Autodesk Fusion 360 part; units mm, degrees
sketch "Excentric Triunghiular Ruleaux + Frame-ul cadrului culisant" plane through (0, 0, 0) normal (1, 0, 0) x (0, 1, 0)
  line L0 (-9.5, 5.4848) -> (0, -10.9697) construction
  line L1 (0, -10.9697) -> (9.5, 5.4848) construction
  line L2 (9.5, 5.4848) -> (-9.5, 5.4848) construction
  arc A0 (0, -10.9697) -> (9.5, 5.4848) centre (-9.5, 5.4848) ccw
  arc A1 (-9.5, 5.4848) -> (0, -10.9697) centre (9.5, 5.4848) ccw
  arc A2 (9.5, 5.4848) -> (-9.5, 5.4848) centre (0, -10.9697) ccw
  circle A3 centre (0, -6) radius 2.5
  line L3 (-17.5, 8.0303) -> (17.5, 8.0303)
  line L4 (17.5, 8.0303) -> (17.5, -10.9697)
  line L5 (17.5, -10.9697) -> (-17.5, -10.9697)
  line L6 (-17.5, -10.9697) -> (-17.5, 8.0303)
  line L7 (0, 8.0303) -> (0, -10.9697) construction
  line L8 (20, -13.4697) -> (-20, -13.4697)
  line L9 (-20, -13.4697) -> (-20, 10.5303)
  line L10 (-20, 10.5303) -> (20, 10.5303)
  line L11 (20, 10.5303) -> (20, -13.4697)
  line L12 (17.5, -1.4697) -> (0, -1.4697) construction
  dimension "d4" = 19
  dimension "d5" = 5
  dimension "d6" = 35
  dimension "d7" = 19
  dimension "d8" = 6
  dimension "d9" = 17.5
  dimension "d10" = -2.5
extrude "Extrude1" add sketch "Excentric Triunghiular Ruleaux + Frame-ul cadrului culisant" along normal blind 5 contours A0 A1 A2
equation "d9 = ( 35 / 2 ) * 1 mm"
Can you work these out from the model? Positions are in its coordinate system, mm. Coordinates: 2 decimals unless noted, no trailing zeros. Loops run counter-clockwise (first coordinate to the right, second up) from the corner with the lowest first, then second, coordinate; pieces in that order, holes last. Notation, with made-up numbers: (53, -9.5) - (68, -9.5) arc R20 cw to (68, 18.5) - close; hole circle Ø6 at (59, 0). An arc over 180 degrees is marked (long way). Answer as CSV lines item,"result". Start each with the question number.
1) Suppose I cut it at B-B (z = -6). Please give me the cut outline in (x, y), plus the area to 3 significant figures.
2) For pin 1 (1 mm diameter, centred on x = 4, z = 0.5, fed in from -Y); pin 2 (1.5 mm diameter, centred on x = 3, z = -3.5, fed in from +Y), each with a flat end and sliding along its axis, tell me the tip position at first contact or that it passes through.
3) Suppose I cut it at D-D (y = -4.25). Please give me the cut outline in (x, z).
4) I need wall thicknesses on line 1 (Z direction, x = 2.8, y = 0.25); line 2 (Z direction, x = 1.1, y = -1); line 3 (Y direction, x = 2.2, z = -4.5). Which ranges of each line are inside material? Lowest first, please. Write a range as from..to.
5) Suppose I cut it at A-A (y = -2). Please give me the cut outline in (x, z), plus the area to 3 significant figures.
6) Suppose I cut it at C-C (x = 4.65). Please give me the cut outline in (y, z), plus the area to 3 significant figures.
7) Thinking about a two-plate mould opening in Y: for faces 1 (the cylindrical face through (2.465, 7.024, -3.894)), 2 (the flat face through (5, 0, 1)), 3 (the cylindrical face through (2.46, -0.33, -8.48)), 4 (the cylindrical face through (2.46, -0.14, 8.03)), which applies, pulls with the +Y half, pulls with the -Y half, needs draft (parallel to the pull), parting line crosses it, or undercut?
Check result:
1,outline,"(0, -5.64) - (5, -5.64) - (5, -2.5) - (0, -2.5) - close; (0, 2.5) - (5, 2.5) - (5, 5.64) - (0, 5.64) - close"
1,area,"31.4 mm²"
2,pin 1,"stops at y = -8.96"
2,pin 2,"stops at y = 7.62"
3,outline,"(0, -7.63) - (5, -7.63) - (5, 7.55) - (0, 7.55) - close"
4,line 1,"z = -10.82..-8.49, -3.51..8.03"
4,line 2,"z = -10.35..-8.29, -3.71..8"
4,line 3,"y = -6.66..-2, 2..6.66"
5,outline,"(0, -9.64) - (5, -9.64) - (5, -7.5) - (0, -7.5) - close; (0, -4.5) - (5, -4.5) - (5, 7.92) - (0, 7.92) - close"
5,area,"72.8 mm²"
6,outline,"(-9.5, 5.48) arc R19 ccw to (0, -10.97) arc R19 ccw to (9.5, 5.48) arc R19 ccw to start; hole circle Ø5 at (0, -6)"
6,area,"235 mm²"
7,face 1,"pulls with the +Y half"
7,face 2,"needs draft"
7,face 3,"undercut"
7,face 4,"parting line crosses it"
